The model under review builds one solid part; all positions refer to its coordinate system, in mm. A direction names the side the tool comes from. Give positions to 0.01 mm unless a question says otherwise; leave off trailing zeros. Order: outer loops, then holes, each group sorted by start corner. A loop starts at its lowest first (then second) coordinate and runs counter-clockwise, first axis right, second up.
```python
from build123d import *

# Parameters (mm, degrees)
SALIENTE_EXTRUIR1_DEPTH = 10
CROQUIS2_R              = 1
CROQUIS2_R_2            = 1.5
CORTAR_EXTRUIR1_DEPTH   = 52.431993934


with BuildPart() as part:
    # Croquis1 → Saliente-Extruir1 (new body)
    with BuildSketch(Plane.XY):
        with BuildLine():
            Line((0, 4), (-15, 4))
            Line((-15, 4), (-15, 8.5))
            Line((-15, 8.5), (0, 8.5))
            ThreePointArc((0, 8.5), (7.288689869, 4.373213921), (7.5, -4))
            Line((7.5, -4), (47.5, -4))
            Line((47.5, -4), (47.5, -8.5))
            Line((47.5, -8.5), (-15, -8.5))
            Line((-15, -8.5), (-15, -4))
            Line((-15, -4), (0, -4))
            ThreePointArc((0, -4), (4, 0), (0, 4))
        make_face()
    extrude(amount=SALIENTE_EXTRUIR1_DEPTH)

    # Croquis2 → Cortar-Extruir1 (cut, through all)
    with BuildSketch(Plane.XZ.offset(8.5)):
        with Locations((42.5, 5)):
            Circle(CROQUIS2_R)
        with Locations((32.5, 5)):
            Circle(CROQUIS2_R)
        with Locations((-8, 5)):
            Circle(CROQUIS2_R_2)
    extrude(amount=-CORTAR_EXTRUIR1_DEPTH, mode=Mode.SUBTRACT)


solid = part.part
```
Item 1: Draft analysis for pull direction Z (two halves, no side actions). For faces 3 (the cylindrical face through (-9.5, -6.28, 5.07)), 4 (the cylindrical face through (43.454, -6.281, 5.3)), 5 (the flat face through (9.5, -4.4, 0)), 6 (the cylindrical face through (4, 0, 5)), state which applies: released by +Z, released by -Z, zero draft, split by the parting line, or undercut.
Values found:
face 3: undercut
face 4: undercut
face 5: released by -Z
face 6: zero draft
Item 2: For faces 1 (the flat face through (9.5, -4.4, 10)), 2 (the flat face through (-6, 4, 5)), list the 3-axis set-ups (+Z, -Z, +X, -X, +Y, -Y) from which the entire face can be reached by the end or side of a thin tool; tool diameter is ignored.
Values found:
face 1: +Z, +X, -X, +Y, -Y
face 2: +Z, -Z, -X
Item 3: Take a section at D-D (x = 42.5). Give the boundary of the cut face in (y, z), and give its area (3 significant figures).
Values found:
outline: (-8.5, 0) - (-4, 0) - (-4, 4) - (-8.5, 4) - close; (-8.5, 6) - (-4, 6) - (-4, 10) - (-8.5, 10) - close
area: 36.0 mm2
Item 4: Take a section at A-A (x = -8). Give the boundary of the cut face in (y, z).
Values found:
outline: (-8.5, 0) - (-4, 0) - (-4, 3.5) - (-8.5, 3.5) - close; (-8.5, 6.5) - (-4, 6.5) - (-4, 10) - (-8.5, 10) - close; (4, 0) - (8.5, 0) - (8.5, 3.5) - (4, 3.5) - close; (4, 6.5) - (8.5, 6.5) - (8.5, 10) - (4, 10) - close
Item 5: For line 1 (Z direction, x = -8, y = 6.3); line 2 (Z direction, x = 32.5, y = -6.3); line 3 (Y direction, x = -8, z = 7), list the stretches that pass through material, from the lowest coordinate up.
Values found:
line 1: z = 0 to 3.5, 6.5 to 10
line 2: z = 0 to 4, 6 to 10
line 3: y = -8.5 to -4, 4 to 8.5
Item 6: Clearance check with flat-ended pins moving along their axes: pin 1 Ø4 at (y, z) = (2.5, 5) entering from +X; pin 2 Ø5 at (y, z) = (4.5, 8) entering from +X. State where each tip first meets the part, or that it passes through.
Values found:
pin 1: stops at x = 8.49
pin 2: stops at x = 8.26
Item 7: Take a section at B-B (y = -6.25). Give the boundary of the cut face in (x, z), and give its area (3 significant figures).
Values found:
outline: (-15, 0) - (47.5, 0) - (47.5, 10) - (-15, 10) - close; hole circle Ø3 at (-8, 5); hole circle Ø2 at (32.5, 5); hole circle Ø2 at (42.5, 5)
area: 612 mm2
Item 8: Take a section at C-C (z = 5). Give the boundary of the cut face in (x, y), and give its area (3 significant figures).
Values found:
outline: (-15, -8.5) - (-9.5, -8.5) - (-9.5, -4) - (-15, -4) - close; (-15, 4) - (-9.5, 4) - (-9.5, 8.5) - (-15, 8.5) - close; (-6.5, -8.5) - (31.5, -8.5) - (31.5, -4) - (7.5, -4) arc R8.5 ccw to (0, 8.5) - (-6.5, 8.5) - (-6.5, 4) - (0, 4) arc R4 cw to (0, -4) - (-6.5, -4) - close; (33.5, -8.5) - (41.5, -8.5) - (41.5, -4) - (33.5, -4) - close; (43.5, -8.5) - (47.5, -8.5) - (47.5, -4) - (43.5, -4) - close
area: 368 mm2
